Design review of the part shown in the three views and the two pictorial views. Dimensions are in mm from the part's minimum x, y and z. Give positions to 0.01 mm unless a question says otherwise; leave off trailing zeros. Loops run counter-clockwise (first coordinate to the right, second up) from the corner with the lowest first, then second, coordinate; pieces in that order, holes last. Notation, with made-up numbers: (22.5, 88) -> (79.5, 88) arc R29 cw to (79.5, 116) -> close; hole circle Ø4 at (-29.5, 64.5). An arc over 180 degrees is marked (long way). Answer as CSV lines item,"result".
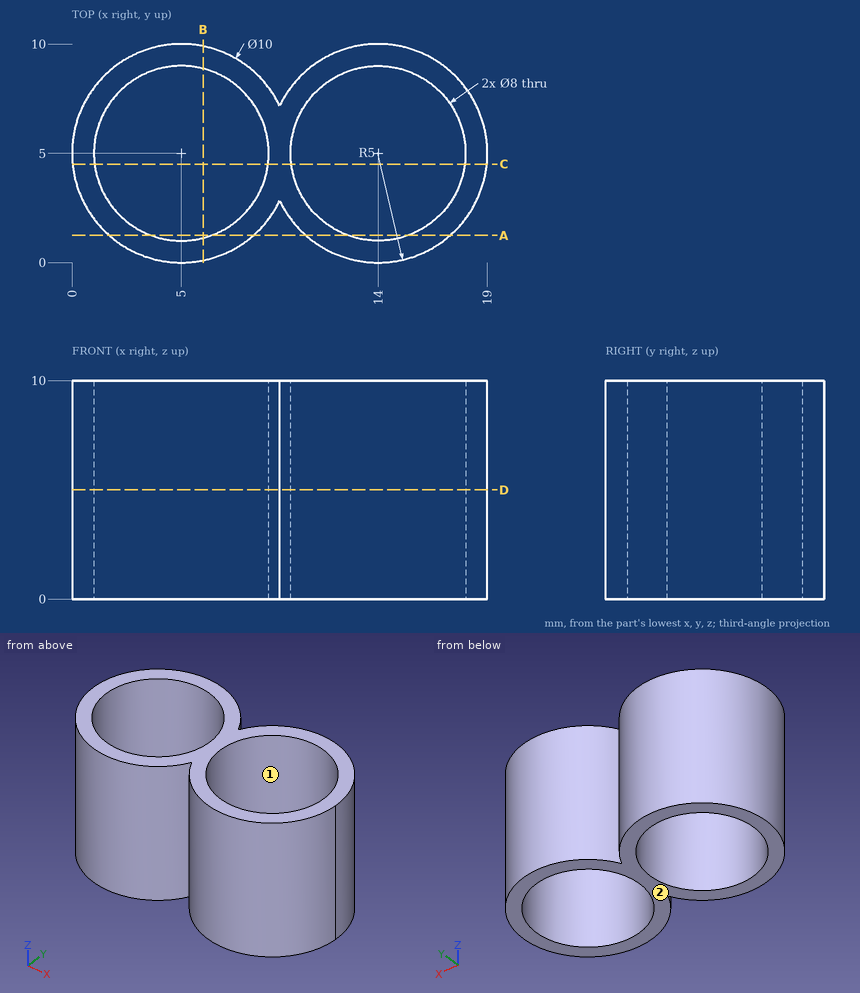
Q1. To check wall thickness, follow probe 1 along Y at (x, z) = (14, 5.75); probe 2 along X at (y, z) = (3.5, 3.5); probe 3 along X at (y, z) = (5.75, 2). State the ranges of each line that lie inside material, in increasing order. Write a range as from..to.
Filled sheet:
probe 1,"y = 0..1, 9..10"
probe 2,"x = 0.23..1.29, 8.71..10.29, 17.71..18.77"
probe 3,"x = 0.06..1.07, 8.93..10.07, 17.93..18.94"
Q2. We need section C-C, the plane y = 4.5. State the section outline as (x, z) points, and give its area (3 significant figures).
Filled sheet:
outline,"(0.03, 0) -> (1.03, 0) -> (1.03, 10) -> (0.03, 10) -> close; (8.97, 0) -> (10.03, 0) -> (10.03, 10) -> (8.97, 10) -> close; (17.97, 0) -> (18.97, 0) -> (18.97, 10) -> (17.97, 10) -> close"
area,"30.8 mm^2"
Q3. Clearance check with flat-ended pins moving along their axes: pin 1 Ø4 at (y, z) = (2, 6.5) entering from +X; pin 2 Ø1 at (y, z) = (9, 7.5) entering from +X. State where each tip first meets the part, or that it passes through.
Filled sheet:
pin 1,"stops at x = 18.9"
pin 2,"stops at x = 17.57"
Q4. We need section D-D, the plane z = 5. State the section outline as (x, y) points.
Filled sheet:
outline,"(9.5, 2.82) arc R5 ccw (long way) to (9.5, 7.18) arc R5 ccw (long way) to start; hole circle Ø8 at (5, 5); hole circle Ø8 at (14, 5)"
Q5. The part is to be moulded in two halves that separate along Y. For the marked faces 1 and 2, say which applies: pulls with the +Y half, pulls with the -Y half, needs draft (parallel to the pull), parting line crosses it, or undercut.
Filled sheet:
face 1,"undercut"
face 2,"needs draft"
Q6. We need section B-B, the plane x = 6. State the section outline as (y, z) points, and give its area (3 significant figures).
Filled sheet:
outline,"(0.1, 0) -> (1.13, 0) -> (1.13, 10) -> (0.1, 10) -> close; (8.87, 0) -> (9.9, 0) -> (9.9, 10) -> (8.87, 10) -> close"
area,"20.5 mm^2"
Q7. We need section A-A, the plane y = 1.25. State the section outline as (x, z) points, and give its area (3 significant figures).
Filled sheet:
outline,"(1.69, 0) -> (3.61, 0) -> (3.61, 10) -> (1.69, 10) -> close; (6.39, 0) -> (8.31, 0) -> (8.31, 10) -> (6.39, 10) -> close; (10.69, 0) -> (12.61, 0) -> (12.61, 10) -> (10.69, 10) -> close; (15.39, 0) -> (17.31, 0) -> (17.31, 10) -> (15.39, 10) -> close"
area,"76.6 mm^2"
